Source: CAD feature listing. Evaluate the final solid. Frame: model axes, mm. Coordinates: 2 decimals unless noted, no trailing zeros. One line per item, written item: value. Start each with the question number.
1. Section query A-A, the plane y = 2.8. State how many separate pieces and enclosed holes the cut face has, and give its area (3 significant figures).
2. Mould query, pull axis X, two halves, no side actions, for faces 1 (the flat face through (-19, 0, 36)), 2 (the cylindrical face through (16.944, 2.218, -3.262)), 3 (the cylindrical face through (-22.08, 2.22, 104.18)). Classes: released by +X, released by -X, zero draft, split by the parting line, or undercut.
3. Line query: line 1 (Z direction, x = -23, y = 2.3); line 2 (X direction, y = 2.3, z = 20); line 3 (X direction, y = 2.2, z = 111). Output: solid intervals per line, ascending.
4. First-contact query: P1, Ø1, axis at x = -21.5, y = 1, coming from the -Z side; P2, Ø1, axis at y = 2, z = 33, coming from the -X side; P3, Ø6.5, axis at x = -23.62, z = 4.48, coming from the -Y side; P4, Ø1.5, axis at y = 3, z = 61.5, coming from the -X side. Flat tips, straight axial feed; report the tip coordinate or a pass-through.
from build123d import *

# Parameters (mm, degrees)
SKETCH1_R           = 1.975
SKETCH1_R_2         = 1.554999938
SKETCH1_R_3         = 0.97
BOSS_EXTRUDE1_DEPTH = 4.5


with BuildPart() as part:
    # Sketch1 → Boss-Extrude1 (new body)
    with BuildSketch(Plane(origin=(0, 0, 0), x_dir=(1, 0, 0), z_dir=(0, 1, 0))):
        with BuildLine():
            Line((-16.144899663, 8.454003274), (10.877745108, 8.454003274))
            ThreePointArc((10.877745108, 8.454003274), (16.961539544, 3.139522495), (12.51277209, -3.603231306))
            ThreePointArc((12.51277209, -3.603231306), (10.56783567, -4.367093581), (8.824099884, -5.518461795))
            add(Edge.make_bspline(
                [(8.824099884, -5.518461795), (4.932532744, -8.718832913), (-4.696045283, -16.58586855), (-31.489086781, -46.943790059), (-12.894682963, -87.326546642), (-17.517744483, -112.138995974)],
                knots=[0.023478108, 0.023478108, 0.023478108, 0.023478108, 0.154944007, 0.330832674, 1, 1, 1, 1], degree=3))
            ThreePointArc((-17.517744483, -112.138995974), (-24.835663445, -118.119615453), (-29.239494185, -109.757437382))
            add(Edge.make_bspline(
                [(-32.217521916, -3.987452131), (-42.206514906, -27.827820505), (-29.561370115, -63.982250345), (-27.390169054, -99.665041987), (-29.239494185, -109.757437382)],
                knots=[0, 0, 0, 0, 0.696305279, 0.977824201, 0.977824201, 0.977824201, 0.977824201], degree=3))
            Line((-32.217521916, -3.987452131), (-16.144899663, 8.454003274))
        make_face()
        with Locations(Location((-23.620555115, -4.478995902, 0), (0, 0, 270))):
            Circle(SKETCH1_R, mode=Mode.SUBTRACT)
        with Locations(Location((-23.620555115, -112.138995974, 0), (0, 0, 270))):
            Circle(SKETCH1_R_2, mode=Mode.SUBTRACT)
        with Locations(Location((-23.620555115, -104.378996, 0), (0, 0, 270))):
            Circle(SKETCH1_R_2, mode=Mode.SUBTRACT)
        with Locations(Location((-23.620555115, -25.918995902, 0), (0, 0, 270))):
            Circle(SKETCH1_R_3, mode=Mode.SUBTRACT)
        with Locations(Location((-23.620555115, -20.098995902, 0), (0, 0, 270))):
            Circle(SKETCH1_R_3, mode=Mode.SUBTRACT)
    extrude(amount=BOSS_EXTRUDE1_DEPTH)


solid = part.part
Computed values:
1. separate pieces: 1
1. enclosed holes: 5
1. area: 2,430 mm²
2. face 1: zero draft
2. face 2: released by +X
2. face 3: undercut
3. line 1: z = -3.15 to 2.6, 6.35 to 19.35, 20.84 to 25.17, 26.66 to 102.95, 105.8 to 110.71, 113.56 to 118.21
3. line 2: x = -36.31 to -24.59, -22.66 to -7.33
3. line 3: x = -29.62 to -24.68, -22.56 to -17.32
4. P1: stops at z = -4.7
4. P2: stops at x = -36.69
4. P3: stops at y = 0
4. P4: stops at x = -32.74
